Could you check a few things on this drawing? It's one solid part, dimensions in mm from its lowest x, y, z. A direction names the side the tool comes from. Coordinates: 2 decimals unless noted, no trailing zeros. Order: outer loops, then holes, each group sorted by start corner. A loop starts at its lowest first (then second) coordinate and runs counter-clockwise, first axis right, second up. Notation, with made-up numbers: (-40, -30.75) - (-23, -30.75) arc R25 ccw to (-23, -18.75) - close; hole circle Ø6 at (76, 22.25). An arc over 180 degrees is marked (long way). Return JSON: item names as keys, results as strings. Group by question number.
1) For pin 1 Ø1.5 at (y, z) = (6.5, 2.5) entering from -X; pin 2 Ø1.5 at (x, z) = (14.5, 4.5) entering from -Y; pin 3 Ø3 at (x, z) = (18, 4) entering from -Y; pin 4 Ø1 at (x, y) = (11.5, 5) entering from +Z, each with a flat end and sliding along its axis, tell me the tip position at first contact or that it passes through.
2) If I drill on line 1 along Z through (x, y) = (20.5, 8); line 2 along Y through (x, z) = (8.75, 4.1); line 3 along Y through (x, z) = (20.25, 0.8), over which ranges is the centre line in solid material (lowest first)?
3) Imagine slicing it at B-B (z = 3.7). Write out the boundary of the cut face in (x, y), and give its area (3 significant figures).
4) Imagine slicing it at A-A (x = 11). Write out the boundary of the cut face in (y, z).
5) Which directions (+Z, -Z, +X, -X, +Y, -Y) give clear straight access to the entire face, cutting with the end or side of a thin tool? Please do the marked faces 1 and 2.
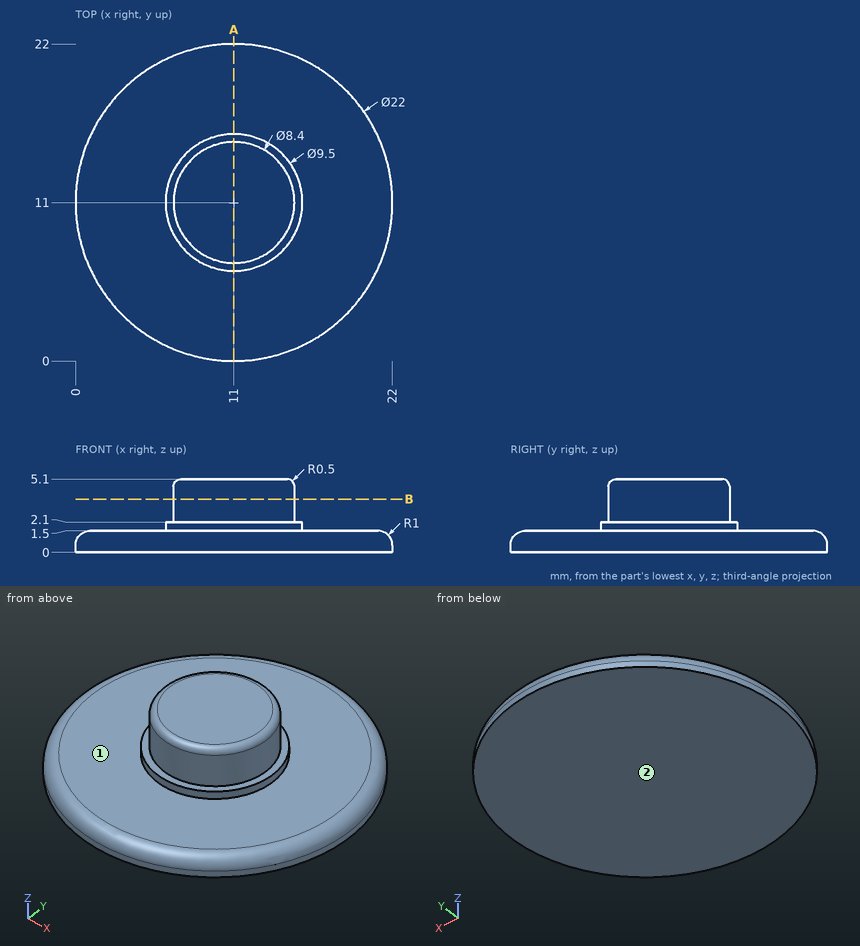
Calculated:
{
 "1": {"pin 1": "x = 8.24", "pin 2": "y = 7.83", "pin 3": "through", "pin 4": "z = 1.5"},
 "2": {"line 1": "0 to 1.5", "line 2": "7.45 to 14.55", "line 3": "5.13 to 16.87"},
 "3": {"outline": "circle Ø8.4 at (11, 11)", "area": "55.4 mm2"},
 "4": {"outline": "(0, 0) - (22, 0) - (22, 0.5) arc R1 ccw to (21, 1.5) - (15.75, 1.5) - (15.75, 2.1) - (15.2, 2.1) - (15.2, 4.6) arc R0.5 ccw to (14.7, 5.1) - (7.3, 5.1) arc R0.5 ccw to (6.8, 4.6) - (6.8, 2.1) - (6.25, 2.1) - (6.25, 1.5) - (1, 1.5) arc R1 ccw to (0, 0.5) - close"},
 "5": {"face 1": "+Z", "face 2": "-Z, +X, -X, +Y, -Y"}
}
